```python
from build123d import *

# Parameters (mm, degrees)
F1_DEPTH = 6.35


with BuildPart() as f1:
    # F0 (on Right) → F1 (new body, symmetric)
    with BuildSketch(Plane.YZ):
        with BuildLine():
            Line((-50.8, 342.9), (-50.8, 0))
            ThreePointArc((-50.8, 0), (0, -50.8), (50.8, 0))
            Line((50.8, 0), (50.8, 342.9))
            ThreePointArc((50.8, 342.9), (0, 393.7), (-50.8, 342.9))
        make_face()
        with BuildLine():
            ThreePointArc((-47.625, 342.9), (0, 390.525), (47.625, 342.9))
            Line((47.625, 342.9), (47.625, 0))
            ThreePointArc((47.625, 0), (0, -47.625), (-47.625, 0))
            Line((-47.625, 0), (-47.625, 342.9))
        make_face(mode=Mode.SUBTRACT)
    extrude(amount=F1_DEPTH, both=True)


solid = f1.part
```
Source: CAD feature listing. Evaluate the final solid. Frame: model axes, mm. A direction names the side the tool comes from. Coordinates: 2 decimals unless noted, no trailing zeros. Write each loop counter-clockwise with the first axis right and the second up, starting at its lowest first coordinate (ties: lowest second). Pieces come first, ordered by that corner, then holes. Notation, with made-up numbers: (66.5, -3.5) - (97.5, -3.5) arc R32 cw to (97.5, 34.5) - close; hole circle Ø5 at (-40, -20.75). An arc over 180 degrees is marked (long way). Answer as a JSON object with one key per item and string values.
Q1. Material intervals for line 1 (Y direction, x = -3.75, z = 41.5) (3 decimals); line 2 (Z direction, x = 1.5, y = 2.5); line 3 (Z direction, x = -4.25, y = 0) (3 decimals), sorted ascending. Write a range as [from, to].
Ans:
{"line 1": "y = [-50.8, -47.625], [47.625, 50.8]", "line 2": "z = [-50.74, -47.56], [390.46, 393.64]", "line 3": "z = [-50.8, -47.625], [390.525, 393.7]"}
Q2. Section query C-C, the plane x = 1.25. Output: boundary loops of the cut face in (y, z) (3 decimals).
Ans:
{"outline": "(-50.8, 0) arc R50.8 ccw to (50.8, 0) - (50.8, 342.9) arc R50.8 ccw to (-50.8, 342.9) - close; hole (-47.625, 0) arc R47.625 ccw to (47.625, 0) - (47.625, 342.9) arc R47.625 ccw to (-47.625, 342.9) - close"}
Q3. Section query B-B, the plane z = 117. Output: boundary loops of the cut face in (x, y) (3 decimals).
Ans:
{"outline": "(-6.35, -50.8) - (6.35, -50.8) - (6.35, -47.625) - (-6.35, -47.625) - close; (-6.35, 47.625) - (6.35, 47.625) - (6.35, 50.8) - (-6.35, 50.8) - close"}
Q4. First-contact query: pin 1 Ø5 at (x, y) = (-2.5, -25) entering from +Z; pin 2 Ø1 at (x, y) = (4, -30) entering from -Z; pin 3 Ø4 at (x, y) = (0.5, -34.5) entering from -Z. Flat tips, straight axial feed; report the tip coordinate or a pass-through.
Ans:
{"pin 1": "stops at z = 388.45", "pin 2": "stops at z = -41.36", "pin 3": "stops at z = -39.04"}
Q5. Section query A-A, the plane y = 0. Output: boundary loops of the cut face in (x, z) (3 decimals).
Ans:
{"outline": "(-6.35, -50.8) - (6.35, -50.8) - (6.35, -47.625) - (-6.35, -47.625) - close; (-6.35, 390.525) - (6.35, 390.525) - (6.35, 393.7) - (-6.35, 393.7) - close"}
Q6. Set-up query: faces 1 (the flat face through (0, -47.625, 169)), 2 (the cylindrical face through (0.089, 1.117, 393.688)). Return all of +Z, -Z, +X, -X, +Y, -Y with unobstructed straight access to the full face (end or side cutting, diameter ignored); none if empty.
Ans:
{"face 1": "+X, -X", "face 2": "+Z, +X, -X"}
Q7. Draft query along Z for faces 3 (the cylindrical face through (0.089, -1.117, -50.788)), 4 (the flat face through (6.35, 49, 172)), 5 (the cylindrical face through (0.089, -1.047, 390.513)). Return one class per face: released by +Z, released by -Z, zero draft, split by the parting line, or undercut.
Ans:
{"face 3": "released by -Z", "face 4": "zero draft", "face 5": "undercut"}
